Could you check a few things on this drawing? It's one solid part, dimensions in mm from its lowest x, y, z. A direction names the side the tool comes from. Give positions to 0.01 mm unless a question says otherwise; leave off trailing zeros. Loops run counter-clockwise (first coordinate to the right, second up) from the corner with the lowest first, then second, coordinate; pieces in that order, holes last. Notation, with made-up numbers: M 60.5,54 L 103.5,54 A29 cw 103.5,87 Z; hole C 62,-25 d2. An arc over 180 degrees is marked long. Answer as a JSON object with one key per item and string values.
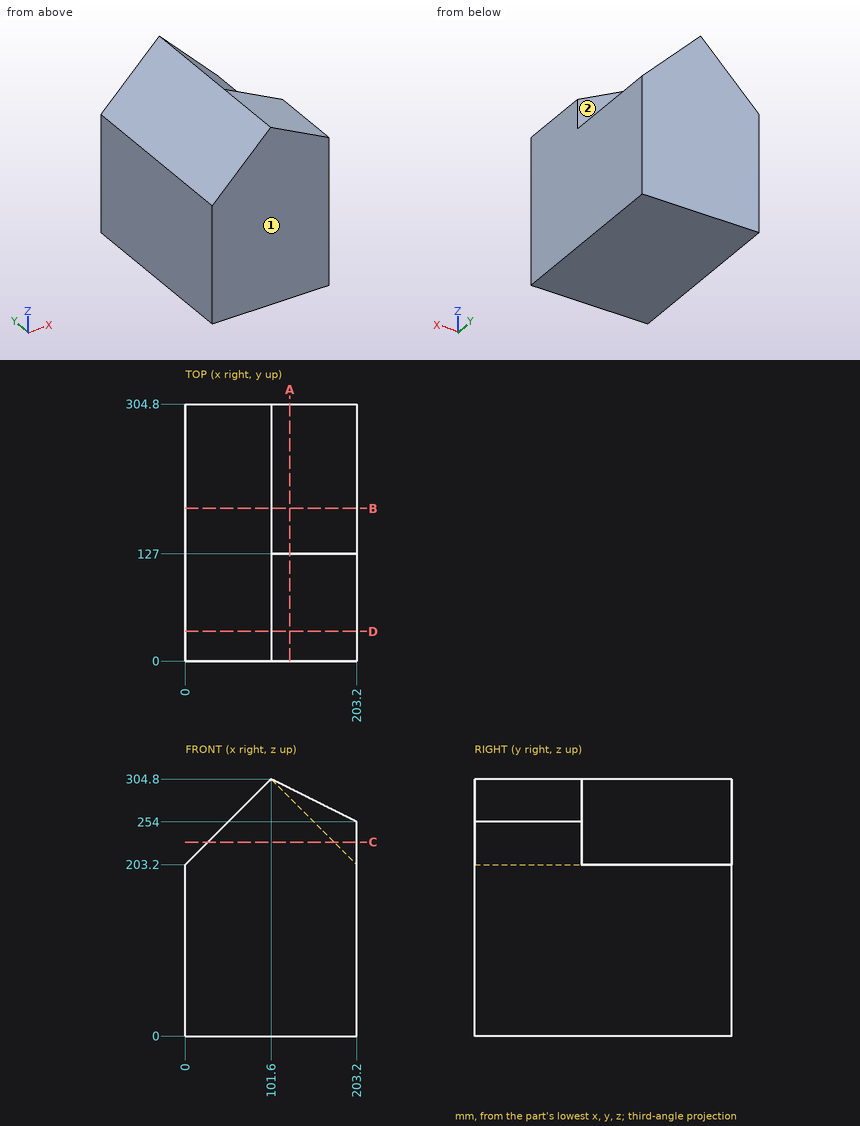
1) Will these pins go through, and if not, where does the flat tip stop? pin 1 Ø10 at (y, z) = (155, 265) entering from -X; pin 2 Ø1 at (x, y) = (74, 174) entering from +Z; pin 3 Ø6 at (x, y) = (75, 247.5) entering from +Z.
Answer list:
{"pin 1": "x = 56.8", "pin 2": "z = 277.7", "pin 3": "z = 281.2"}
2) Suppose I cut it at B-B, the plane y = 181. Write out the boundary of the cut face in (x, z).
Answer list:
{"outline": "M 0,0 L 203.2,0 L 203.2,203.2 L 101.6,304.8 L 0,203.2 Z"}
3) Please list where these lines run through material, in increasing order: line 1 along Z through (x, y) = (71.5, 244); line 2 along Z through (x, y) = (69.5, 31); line 3 along X through (y, z) = (114, 255.5). Write a range as from..to.
Answer list:
{"line 1": "0..274.7", "line 2": "0..272.7", "line 3": "52.3..200.2"}
4) Suppose I cut it at D-D, the plane y = 35. Write out the boundary of the cut face in (x, z), and give its area (3 significant figures).
Answer list:
{"outline": "M 0,0 L 203.2,0 L 203.2,254 L 101.6,304.8 L 0,203.2 Z", "area": "54,200 mm^2"}
5) Suppose I cut it at A-A, the plane x = 124. Write out the boundary of the cut face in (y, z), and give its area (3 significant figures).
Answer list:
{"outline": "M 0,0 L 304.8,0 L 304.8,282.4 L 127,282.4 L 127,293.6 L 0,293.6 Z", "area": "87,500 mm^2"}
6) Suppose I cut it at C-C, the plane z = 230. Write out the boundary of the cut face in (x, y), and give its area (3 significant figures).
Answer list:
{"outline": "M 26.8,0 L 203.2,0 L 203.2,127 L 176.4,127 L 176.4,304.8 L 26.8,304.8 Z", "area": "49,000 mm^2"}
7) For the marked faces 1 and 2, which set-ups out of +Z, -Z, +X, -X, +Y, -Y let a thin tool reach every point of the face, with its end or its side?
Answer list:
{"face 1": "+Z, -Z, +X, -X, -Y", "face 2": "+Z, +X, +Y"}
